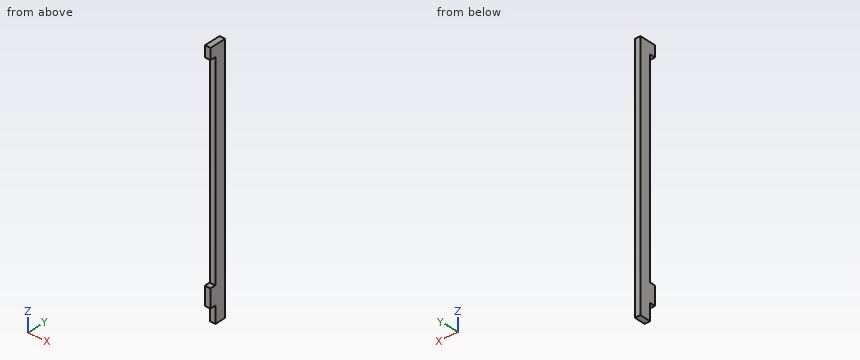
```python
from build123d import *

# Parameters (mm, degrees)
EXTRUDE_START            = -274
SKETCH_1_W               = 6
SKETCH_1_H               = 12
EXTRUDE_1_DEPTH          = 268
CUT_EXTRUDE_2_DEPTH      = 335.505178406
CUT_EXTRUDE_2_DEPTH_BACK = 335.505178406
SKETCH_3106_W            = 6
SKETCH_3106_H            = 6.1
EXTRUDE_3215_DEPTH       = 6
OTHER_START              = 57.8
OTHER_3265_OUTLINE_W     = 6
OTHER_3265_OUTLINE_H     = 6
OTHER_3265_DEPTH         = 5.8
SKETCH_3419_W            = 24
SKETCH_3419_H            = 12
EXTRUDE_3519_DEPTH       = 6
OTHER_START_2            = -176.272727273
OTHER_3590_OUTLINE_W     = 6
OTHER_3590_OUTLINE_H     = 20
OTHER_3590_DEPTH         = 6
SKETCH_2_W               = 6
SKETCH_2_H               = 12.2
EXTRUDE_2_DEPTH          = 6


# Read off the part's stored shape, not the designer's step: the other step, the other step
with BuildPart() as part:
    # Sketch 1 → Extrude 1 (new body)
    with BuildSketch(Plane.XY.offset(EXTRUDE_START)):
        with Locations((-173.272727273, 69.8)):
            Rectangle(SKETCH_1_W, SKETCH_1_H)
    extrude(amount=EXTRUDE_1_DEPTH)

    # Sketch 3011 → Cut-Extrude 2 (cut, two sides: drawn at the far end of the back side and taken through both)
    with BuildSketch(Plane(origin=(0, 0, 0), x_dir=(0, 0, -1), z_dir=(1, 0, 0)).offset(-CUT_EXTRUDE_2_DEPTH_BACK)):
        Polygon((140.075, 62.8), (139.925, 62.8), (139.925, 66.725), (127.925, 66.725), (127.925, 72.875), (139.925, 72.875), (139.925, 76.8), (140.075, 76.8), (140.075, 72.725), (128.075, 72.725), (128.075, 66.875), (140.075, 66.875), align=None)
    extrude(amount=CUT_EXTRUDE_2_DEPTH + CUT_EXTRUDE_2_DEPTH_BACK, mode=Mode.SUBTRACT)


with BuildPart() as cut_extrude_2_piece_1:
    # of the separate pieces the step leaves, piece 1, a body of its own (cut_extrude_2_pieces)
    add(part.part.solids().sort_by_distance((-176.272727273, 75.8, -274))[0])



with BuildPart() as cut_extrude_2_piece_2:
    # of the separate pieces the step leaves, piece 2, a body of its own (cut_extrude_2_pieces)
    add(part.part.solids().sort_by_distance((-176.272727273, 75.8, -139.925))[0])

    # Sketch 3106 → Extrude 3215 (add)
    with BuildSketch(Plane.ZY.offset(176.272727273)):
        with Locations((-9, 60.85)):
            Rectangle(SKETCH_3106_W, SKETCH_3106_H)
    extrude(amount=-EXTRUDE_3215_DEPTH)

    # Other 3265 outline → Other 3265 (add)
    with BuildSketch(Plane(origin=(0, 0, 0), x_dir=(1, 0, 0), z_dir=(0, 1, 0)).offset(OTHER_START)):
        with Locations((-173.272727273, 3)):
            Rectangle(OTHER_3265_OUTLINE_W, OTHER_3265_OUTLINE_H)
    extrude(amount=OTHER_3265_DEPTH)


with BuildPart() as cut_extrude_2_piece_1_1:
    add(cut_extrude_2_piece_1.part)

    add(cut_extrude_2_piece_2.part)  # Extrude 3519 merges Cut-Extrude 2 piece 2
    # Sketch 3419 → Extrude 3519 (add)
    with BuildSketch(Plane.ZY.offset(176.272727273)):
        with Locations((-134, 69.8)):
            Rectangle(SKETCH_3419_W, SKETCH_3419_H)
    extrude(amount=-EXTRUDE_3519_DEPTH)

    # Other 3590 outline → Other 3590 (add)
    with BuildSketch(Plane.YZ.offset(OTHER_START_2)):
        with Locations((60.8, -246)):
            Rectangle(OTHER_3590_OUTLINE_W, OTHER_3590_OUTLINE_H)
    extrude(amount=OTHER_3590_DEPTH)

    # Sketch 2 → Extrude 2 (add)
    with BuildSketch(Plane.XY.offset(-6)):
        with Locations((-173.272727273, 69.7)):
            Rectangle(SKETCH_2_W, SKETCH_2_H)
    extrude(amount=EXTRUDE_2_DEPTH)


solid = cut_extrude_2_piece_1_1.part
```
Design review of the part built by this model. Coordinates are the model's own, in mm. Round coordinates to 2 decimals unless told otherwise and drop trailing zeros. Write each loop counter-clockwise with the first axis right and the second up, starting at its lowest first coordinate (ties: lowest second). Pieces come first, ordered by that corner, then holes. Notation, with made-up numbers: (36, -29) -> (46, -29) arc R22 ccw to (46, -7) -> close; hole circle Ø5 at (16, 62). An arc over 180 degrees is marked (long way). Answer in a Markdown table with one row per item.
Q1. Take a section at A-A, the plane x = -173.1. State the section outline as (y, z) points, then the cut area to 3 significant figures.
The answers:
| item | result |
|---|---|
| outline | (57.8, -256) -> (63.8, -256) -> (63.8, -274) -> (75.8, -274) -> (75.8, 0) -> (57.8, 0) -> (57.8, -12) -> (63.8, -12) -> (63.8, -236) -> (57.8, -236) -> close |
| area | 3,480 mm² |
Q2. Clearance check with a flat-ended pin moving along its axis: pin 1 Ø1.8 at (x, z) = (-174, -265) entering from -Y. State where the tip first meets the part, or that it passes through.
The answers:
| item | result |
|---|---|
| pin 1 | y = 63.8 |
Q3. To check wall thickness, follow L1, parallel to Z at x = -175, y = 60; L2, parallel to Y at x = -171, z = -80. State the ranges of each line that lie inside material, in increasing order. Write a range as [from, to].
The answers:
| item | result |
|---|---|
| L1 | [-256, -236], [-12, 0] |
| L2 | [63.8, 75.8] |
Q4. Take a section at B-B, the plane z = -30. State the section outline as (x, y) points, then the cut area to 3 significant figures.
The answers:
| item | result |
|---|---|
| outline | (-176.27, 63.8) -> (-170.27, 63.8) -> (-170.27, 75.8) -> (-176.27, 75.8) -> close |
| area | 72.0 mm² |
